from build123d import *

# Parameters (mm, degrees)
SKETCH_1_R               = 6
EXTRUDE_1_DEPTH          = 19
SKETCH_2_R               = 1.5
CUT_EXTRUDE_1_DEPTH      = 9.5
SKETCH_3_W               = 13.627836578
SKETCH_3_H               = 1
CUT_EXTRUDE_2_DEPTH      = 6
SKETCH_4_W               = 1
SKETCH_4_H               = 12.796097453
CUT_EXTRUDE_3_DEPTH      = 6
CUT_EXTRUDE_5_DEPTH      = 6
CUT_EXTRUDE_5_DEPTH_BACK = 6
SKETCH_5_R               = 1
CUT_EXTRUDE_START        = -2
SKETCH_6_R               = 1.5
CUT_EXTRUDE_6_DEPTH      = 6
SKETCH_7_R               = 1
CUT_EXTRUDE_7_DEPTH      = 6
SKETCH_8_R               = 1.5
CUT_EXTRUDE_8_DEPTH      = 6
SKETCH_9_R               = 2
CUT_EXTRUDE_9_DEPTH      = 9.5


with BuildPart() as part:
    # 草图1 → 凸台-拉伸1 (new body)
    with BuildSketch(Plane.XY):
        Circle(SKETCH_1_R)
    extrude(amount=EXTRUDE_1_DEPTH)

    # 草图2 → 切除-拉伸1 (cut)
    with BuildSketch(Plane.XY.offset(19)):
        Circle(SKETCH_2_R)
    extrude(amount=-CUT_EXTRUDE_1_DEPTH, mode=Mode.SUBTRACT)

    # 草图3 → 切除-拉伸2 (cut)
    with BuildSketch(Plane.XY.offset(19)):
        with Locations((-0.190601878, 0)):
            Rectangle(SKETCH_3_W, SKETCH_3_H)
    extrude(amount=-CUT_EXTRUDE_2_DEPTH, mode=Mode.SUBTRACT)

    # 草图4 → 切除-拉伸3 (cut)
    with BuildSketch(Plane(origin=(0, 0, 0), x_dir=(-1, 0, 0), z_dir=(0, 0, -1))):
        with Locations((0, -0.108476873)):
            Rectangle(SKETCH_4_W, SKETCH_4_H)
    extrude(amount=-CUT_EXTRUDE_3_DEPTH, mode=Mode.SUBTRACT)

    # 草图5 → 切除-拉伸5 (cut, two sides: drawn at the far end of the back side and taken through both)
    with BuildSketch(Plane(origin=(0, 0, 0), x_dir=(1, 0, 0), z_dir=(0, 1, 0)).offset(-CUT_EXTRUDE_5_DEPTH_BACK)):
        with Locations(Location((-4, -16, 0), (0, 0, 90))):
            Circle(SKETCH_5_R)
        with Locations(Location((4, -16, 0), (0, 0, 90))):
            Circle(SKETCH_5_R)
    extrude(amount=CUT_EXTRUDE_5_DEPTH + CUT_EXTRUDE_5_DEPTH_BACK, mode=Mode.SUBTRACT)

    # 草图6 → 切除-拉伸6 (cut)
    with BuildSketch(Plane(origin=(0, 0, 0), x_dir=(1, 0, 0), z_dir=(0, 1, 0)).offset(CUT_EXTRUDE_START)):
        with Locations(Location((-4, -16, 0), (0, 0, 270))):
            Circle(SKETCH_6_R)
        with Locations(Location((4, -16, 0), (0, 0, 270))):
            Circle(SKETCH_6_R)
    cut_extrude_6 = extrude(amount=-CUT_EXTRUDE_6_DEPTH, mode=Mode.SUBTRACT)

    # 镜向1: 切除-拉伸6 across plane
    add(cut_extrude_6.mirror(Plane.ZX), mode=Mode.SUBTRACT)

    # 草图7 → 切除-拉伸7 (cut)
    with BuildSketch(Plane(origin=(0, 0, 0), x_dir=(0, 0, -1), z_dir=(1, 0, 0))):
        with Locations((-3, 4)):
            Circle(SKETCH_7_R)
        with Locations((-3, -4)):
            Circle(SKETCH_7_R)
    cut_extrude_7 = extrude(amount=-CUT_EXTRUDE_7_DEPTH, mode=Mode.SUBTRACT)

    # 草图8 → 切除-拉伸8 (cut)
    with BuildSketch(Plane(origin=(0, 0, 0), x_dir=(0, 0, -1), z_dir=(1, 0, 0)).offset(CUT_EXTRUDE_START)):
        with Locations((-3, -4)):
            Circle(SKETCH_8_R)
        with Locations((-3, 4)):
            Circle(SKETCH_8_R)
    cut_extrude_8 = extrude(amount=-CUT_EXTRUDE_8_DEPTH, mode=Mode.SUBTRACT)

    # 镜向2: 切除-拉伸7, 切除-拉伸8 across plane
    add(cut_extrude_7.mirror(Plane(origin=(0, 0, 0), x_dir=(0, 0, 1), z_dir=(1, 0, 0))), mode=Mode.SUBTRACT)
    add(cut_extrude_8.mirror(Plane(origin=(0, 0, 0), x_dir=(0, 0, 1), z_dir=(1, 0, 0))), mode=Mode.SUBTRACT)

    # 草图9 → 切除-拉伸9 (cut)
    with BuildSketch(Plane(origin=(0, 0, 0), x_dir=(-1, 0, 0), z_dir=(0, 0, -1))):
        Circle(SKETCH_9_R)
    extrude(amount=-CUT_EXTRUDE_9_DEPTH, mode=Mode.SUBTRACT)


solid = part.part
Could you check a few things on this model? Use its own coordinates, in mm. A direction names the side the tool comes from. Give positions to 0.01 mm unless a question says otherwise; leave off trailing zeros. Order: outer loops, then holes, each group sorted by start corner. A loop starts at its lowest first (then second) coordinate and runs counter-clockwise, first axis right, second up.
Item 1: I'm going to push flat-ended pins straight in: pin 1 (0.5 mm diameter, centred on x = 0, y = -4.5, fed in from -Z); pin 2 (2.5 mm diameter, centred on x = 4.5, z = 15.5, fed in from +Y); pin 3 (0.8 mm diameter, centred on x = 5, y = 0, fed in from +Z); pin 4 (1.8 mm diameter, centred on y = -4, z = 3, fed in from +X). Where does each tip first touch, or does it pass through?
Item 2: If we mould it in two halves opening along Z, with no side actions, what happens to faces 1 (the face through (-0.5, -3, 2)), 2 (the face through (0, 3, 19)), 3 (the face through (-3.319, -2.513, 3.195)), 4 (the face through (3.319, -2.513, 3.195))? For each: pulls with the +Z half, pulls with the -Z half, needs draft (parallel to the pull), parting line crosses it, or undercut.
Item 3: If we section it at C-C, the plane y = 0: Write out the boundary of the cut face in (x, z), plus the area to 4 significant figures.
Item 4: If we section it at D-D, the plane y = -4: Write out the boundary of the cut face in (x, z), plus the area to 3 significant figures.
Item 5: For faces 5 (the face through (0.5, 5, 2)), 6 (the face through (3, -0.5, 15)), 7 (the face through (3.319, 2.536, 3.325)), which set-ups out of +Z, -Z, +X, -X, +Y, -Y let a thin tool reach every point of the face, with its end or its side?
Item 6: If we section it at B-B, the plane x = 0: Write out the boundary of the cut face in (y, z), plus the area to 4 significant figures.
Item 7: I need wall thicknesses on line 1 (Y direction, x = 1.35, z = 3); line 2 (X direction, y = -0.5, z = 3); line 3 (Z direction, x = 4.25, y = 3). Which ranges of each line are inside material? Lowest first, please.
Item 8: If we section it at A-A, the plane z = 14.25: Write out the boundary of the cut face in (x, y), plus the area to 3 significant figures.
Values:
1. pin 1: stops at z = 6
1. pin 2: stops at y = 4.71
1. pin 3: stops at z = 13
1. pin 4: passes through
2. face 1: needs draft
2. face 2: pulls with the +Z half
2. face 3: undercut
2. face 4: undercut
3. outline: (-6, 0) - (-2, 0) - (-2, 9.5) - (-1.5, 9.5) - (-1.5, 13) - (-6, 13) - close; (1.5, 9.5) - (2, 9.5) - (2, 0) - (6, 0) - (6, 13) - (1.5, 13) - close
3. area: 107.5 mm2
4. outline: (-4.47, 0) - (-0.5, 0) - (-0.5, 2) - (-2, 2) - (-2, 1.5) - (-4.47, 1.5) - close; (-4.47, 4.5) - (-2, 4.5) - (-2, 4) - (-0.5, 4) - (-0.5, 6) - (0.5, 6) - (0.5, 4) - (2, 4) - (2, 4.5) - (4.47, 4.5) - (4.47, 14.58) arc R1.5 cw (long way) to (4.47, 17.42) - (4.47, 19) - (-4.47, 19) - (-4.47, 17.42) arc R1.5 cw (long way) to (-4.47, 14.58) - close; (0.5, 0) - (4.47, 0) - (4.47, 1.5) - (2, 1.5) - (2, 2) - (0.5, 2) - close
4. area: 133 mm2
5. face 5: -Z, +Y, -Y
5. face 6: +Z, +X, -X
5. face 7: +X
6. outline: (-6, 6) - (-2, 6) - (-2, 9.5) - (-1.5, 9.5) - (-1.5, 19) - (-6, 19) - close; (1.5, 9.5) - (2, 9.5) - (2, 6) - (6, 6) - (6, 19) - (1.5, 19) - close
6. area: 113.5 mm2
7. line 1: y = -5.85 to -5, -3 to -1.48, 1.48 to 3, 5 to 5.85
7. line 2: x = -5.98 to -1.94, 1.94 to 5.98
7. line 3: z = 0 to 1.88, 4.12 to 14.52, 17.48 to 19
8. outline: (-5.98, -0.5) arc R6 ccw to (5.98, -0.5) - (1.41, -0.5) arc R1.5 cw to (-1.41, -0.5) - close; (-5.98, 0.5) - (-1.41, 0.5) arc R1.5 cw to (1.41, 0.5) - (5.98, 0.5) arc R6 ccw to start
8. area: 97.0 mm2
